Here's how the part is built. I have some questions about the finished solid (model axes, mm). A direction names the side the tool comes from. Round coordinates to 2 decimals unless told otherwise and drop trailing zeros. Loops run counter-clockwise (first coordinate to the right, second up) from the corner with the lowest first, then second, coordinate; pieces in that order, holes last. Notation, with made-up numbers: M -33,43 L 20,43 A22 cw 20,62 Z; hole C 50,73 d8. An arc over 180 degrees is marked long. Put each result on its own line as item: value. Start each with the question number.
```python
from build123d import *
from OCP.BRepFilletAPI import BRepFilletAPI_MakeChamfer

# Parameters (mm, degrees)
SKETCH_1_R          = 2.1
EXTRUDE_1_DEPTH     = 2.5
CUT_EXTRUDE_1_DEPTH = 95.372930441
EXTRUDE_2_DEPTH     = 5
CUT_EXTRUDE_2_DEPTH = 142.00635371
FILLET_1_R          = 5
FILLET_2_R          = 4
FILLET_3_R          = 15
CHAMFER_1_SIZE      = 4
CHAMFER_1_SIZE2     = 6.20437999
CHAMFER_2_SIZE      = 2
SKETCH_6_R          = 3.1
CUT_EXTRUDE_3_DEPTH = 140.696602049
CUT_EXTRUDE_4_DEPTH = 140.696602049
CHAMFER_3_SIZE      = 3
FILLET_4_R          = 1


with BuildPart() as part:
    # 草图1 → 凸台-拉伸1 (new, symmetric)
    with BuildSketch(Plane.XY):
        Polygon((-35, 87.5), (-35, -87.5), (35, -87.5), (35, -67.5), (-15, 87.5), align=None)
        with Locations((-25, -77.5)):
            Circle(SKETCH_1_R, mode=Mode.SUBTRACT)
        with Locations((25, -77.5)):
            Circle(SKETCH_1_R, mode=Mode.SUBTRACT)
        with Locations((-25, 77.5)):
            Circle(SKETCH_1_R, mode=Mode.SUBTRACT)
        with Locations((-25, -57.5)):
            Circle(SKETCH_1_R, mode=Mode.SUBTRACT)
    extrude(amount=EXTRUDE_1_DEPTH, both=True)

    # 草图2 → 切除-拉伸1 (cut, through all)
    with BuildSketch(Plane(origin=(0, 0, -2.5), x_dir=(-1, 0, 0), z_dir=(0, 0, -1))):
        with BuildLine():
            Line((-17.130804412, -60.9649861), (5.241456911, 8.389024))
            ThreePointArc((5.241456911, 8.389024), (11.5350139, 11.612553189), (14.758543089, 5.318996201))
            Line((14.758543089, 5.318996201), (-7.613718234, -64.0350139))
            ThreePointArc((-7.613718234, -64.0350139), (-13.907275222, -67.258543089), (-17.130804412, -60.9649861))
        make_face()
    extrude(amount=-CUT_EXTRUDE_1_DEPTH, mode=Mode.SUBTRACT)

    # 草图3 → 凸台-拉伸2 (add)
    with BuildSketch(Plane(origin=(0, 0, -2.5), x_dir=(-1, 0, 0), z_dir=(0, 0, -1))):
        Polygon((35, -87.5), (92.302946454, -84.303295451), (110.460589291, -75.918785529), (35, 87.5), align=None)
    extrude(amount=-EXTRUDE_2_DEPTH)

    # 草图5 → 切除-拉伸2 (cut, through all)
    with BuildSketch(Plane(origin=(0, 0, -2.5), x_dir=(-1, 0, 0), z_dir=(0, 0, -1))):
        Polygon((35, 39.792977913), (58.598142626, -11.311576727), (35, -65.049025296), align=None)
        Polygon((87.794289034, -74.539267276), (40.598003783, -77.172161204), (64.196146409, -23.434712635), align=None)
    extrude(amount=-CUT_EXTRUDE_2_DEPTH, mode=Mode.SUBTRACT)

    # 圆角1
    fillet_1_edges = [part.edges().sort_by_distance(p)[0] for p in [
        (-64.196146409, -23.434712635, 0),
        (-87.794289034, -74.539267276, 0),
        (-40.598003783, -77.172161204, 0),
        (-35, 39.792977913, 0),
    ]]
    fillet(fillet_1_edges, radius=FILLET_1_R)

    # 圆角2
    fillet_2_edges = [part.edges().sort_by_distance(p)[0] for p in [
        (-35, -65.049025296, 0),
    ]]
    fillet(fillet_2_edges, radius=FILLET_2_R)

    # 圆角3
    fillet_3_edges = [part.edges().sort_by_distance(p)[0] for p in [
        (-58.598142626, -11.311576727, 0),
    ]]
    fillet(fillet_3_edges, radius=FILLET_3_R)

    # 倒角1: one chamfer whose edges measure the first distance from different faces: ONE call of the kernel's chamfer builder (chamfer() names one face for all edges)
    chamfer_1_edges_1 = [part.edges().sort_by_distance(p)[0] for p in [
        (-110.460589291, -75.918785529, 0),
        (35, -87.5, 0),
    ]]
    chamfer_1_edges_2 = [part.edges().sort_by_distance(p)[0] for p in [
        (-15, 87.5, 0),
    ]]
    chamfer_1_side_2 = [part.faces().sort_by_distance(p)[0] for p in [
        (-25, 87.5, 0),
    ]]
    chamfer_1 = BRepFilletAPI_MakeChamfer(part.part.solid().wrapped)
    for e in chamfer_1_edges_1:
        chamfer_1.Add(CHAMFER_1_SIZE, e.wrapped)
    for e in chamfer_1_edges_2:
        chamfer_1.Add(CHAMFER_1_SIZE, CHAMFER_1_SIZE2, e.wrapped, chamfer_1_side_2[0].wrapped)  # the first distance lies on this face
    add(Compound.cast(chamfer_1.Shape()), mode=Mode.REPLACE)

    # 倒角2
    chamfer_2_edges = [part.edges().sort_by_distance(p)[0] for p in [
        (22.9, -77.5, 2.5),
        (-27.1, -77.5, 2.5),
        (-27.1, 77.5, 2.5),
        (-27.1, -57.5, 2.5),
    ]]
    chamfer(chamfer_2_edges, length=CHAMFER_2_SIZE)

    # 草图6 → 切除-拉伸3 (cut, through all)
    with BuildSketch(Plane(origin=(0, 0, -2.5), x_dir=(-1, 0, 0), z_dir=(0, 0, -1))):
        with Locations((97.189512912, -71.032219072)):
            Circle(SKETCH_6_R)
        with Locations((44.786325904, 42.453048657)):
            Circle(SKETCH_6_R)
    extrude(amount=-CUT_EXTRUDE_3_DEPTH, mode=Mode.SUBTRACT)

    # 草图7 → 切除-拉伸4 (cut, through all)
    with BuildSketch(Plane.XY.offset(2.5)):
        Polygon((-58.057402283, 37.566482199), (-53.170835826, 24.29540582), (-88.805002991, -52.874576235), (-102.07607937, -57.761142693), align=None)
    extrude(amount=-CUT_EXTRUDE_4_DEPTH, mode=Mode.SUBTRACT)

    # 倒角3
    chamfer_3_edges = [part.edges().sort_by_distance(p)[0] for p in [
        (-94.089512912, -71.032219072, -2.5),
        (-41.686325904, 42.453048657, -2.5),
    ]]
    chamfer(chamfer_3_edges, length=CHAMFER_3_SIZE)

    # 圆角4
    fillet_4_edges = [part.edges().sort_by_distance(p)[0] for p in [
        (-53.170835826, 24.29540582, 0),
        (-88.805002991, -52.874576235, 0),
    ]]
    fillet(fillet_4_edges, radius=FILLET_4_R)


solid = part.part
```
1) If we mould it in two halves opening along X, with no side actions, what happens to faces 1 (the face through (-46.531, 45.19, 0.354)), 2 (the face through (-55.72, 31.22, 0.04)), 3 (the face through (-20, -18, 2.5))? For each: pulls with the +X half, pulls with the -X half, needs draft (parallel to the pull), parting line crosses it, or undercut.
2) Suppose I cut it at C-C (y = -41). Write out the boundary of the cut face in (x, z), plus the area to 3 significant figures.
3) Suppose I cut it at A-A (x = 25). Write out the boundary of the cut face in (y, z), plus the area to 3 significant figures.
4) On a 3-axis mill with a long thin cutter (end or side, diameter ignored), from which of +Z, -Z, +X, -X, +Y, -Y can I reach the whole of each face in a straight line? I mean faces 4 (the face through (-25.482, -59.672, 0.625)), 5 (the face through (-50.074, 7.148, -0.035)). Say none if no direction works.
5) If I drill on probe 1 along Y at (x, z) = (-25, -1.2); probe 2 along X at (y, z) = (-66, 0.9); probe 3 along X at (y, z) = (-40, 1.6), over which ranges is the centre line in solid material (lowest first)? Write a range as from..to.
6) Suppose I cut it at D-D (z = 1.3). State how many separate pieces and enclosed holes the cut face has, plus the area to 3 significant figures.
7) I'm going to push flat-ended pins straight in: P1, Ø6.5, axis at x = 25, y = -77.5, coming from the +Z side; P2, Ø2, axis at x = -44, z = 0, coming from the -Y side; P3, Ø10, axis at x = -97.19, y = -71.03, coming from the -Z side. Where does each tip first touch, or does it pass through?
8) Suppose I cut it at B-B (x = -25). Write out the boundary of the cut face in (y, z).
Results are:
1. face 1: undercut
1. face 2: pulls with the -X half
1. face 3: needs draft
2. outline: M -83.32,-2.5 L -72.31,-2.5 L -72.31,2.5 L -83.32,2.5 Z; M -56.48,-2.5 L -45.56,-2.5 L -45.56,2.5 L -56.48,2.5 Z; M -35,-2.5 L 0.18,-2.5 L 0.18,2.5 L -35,2.5 Z; M 10.69,-2.5 L 26.45,-2.5 L 26.45,2.5 L 10.69,2.5 Z
2. area: 364 mm²
3. outline: M -87.5,-2.5 L -79.6,-2.5 L -79.6,0.5 L -81.6,2.5 L -87.5,2.5 Z; M -75.4,-2.5 L -36.5,-2.5 L -36.5,2.5 L -73.4,2.5 L -75.4,0.5 Z
3. area: 230 mm²
4. face 4: +Z
4. face 5: +Z, -Z
5. probe 1: -87.5..-79.6, -75.4..-59.6, -55.4..75.4, 79.6..87.5
5. probe 2: -105.88..-83.85, -45.5..8.8, 15.94..34.52
5. probe 3: -82.86..-71.85, -56.92..-46, -35..-0.14, 10.37..26.13
6. separate pieces: 1
6. enclosed holes: 9
6. area: 11,000 mm²
7. P1: z = 1.65
7. P2: y = -87.05
7. P3: z = -1.4
8. outline: M -87.5,-2.5 L -79.6,-2.5 L -79.6,0.5 L -81.6,2.5 L -87.5,2.5 Z; M -75.4,-2.5 L -59.6,-2.5 L -59.6,0.5 L -61.6,2.5 L -73.4,2.5 L -75.4,0.5 Z; M -55.4,-2.5 L 75.4,-2.5 L 75.4,0.5 L 73.4,2.5 L -53.4,2.5 L -55.4,0.5 Z; M 79.6,-2.5 L 87.5,-2.5 L 87.5,2.5 L 81.6,2.5 L 79.6,0.5 Z
